Study the drawing (mm; zero at the part's minimum x, y, z) and answer. A direction names the side the tool comes from. Give positions to 0.01 mm unless a question says otherwise; leave off trailing zeros. Write each loop counter-clockwise with the first axis right and the second up, starting at its lowest first coordinate (ties: lowest second). Pieces come first, ordered by that corner, then holes. Notation, with made-up numbers: (-20, 42) -> (-16, 42) arc R18 ccw to (-16, 68) -> close; hole circle Ø6 at (15, -3.5). An arc over 180 degrees is marked (long way). Put each result on its own line as item: value. Start each with the question number.
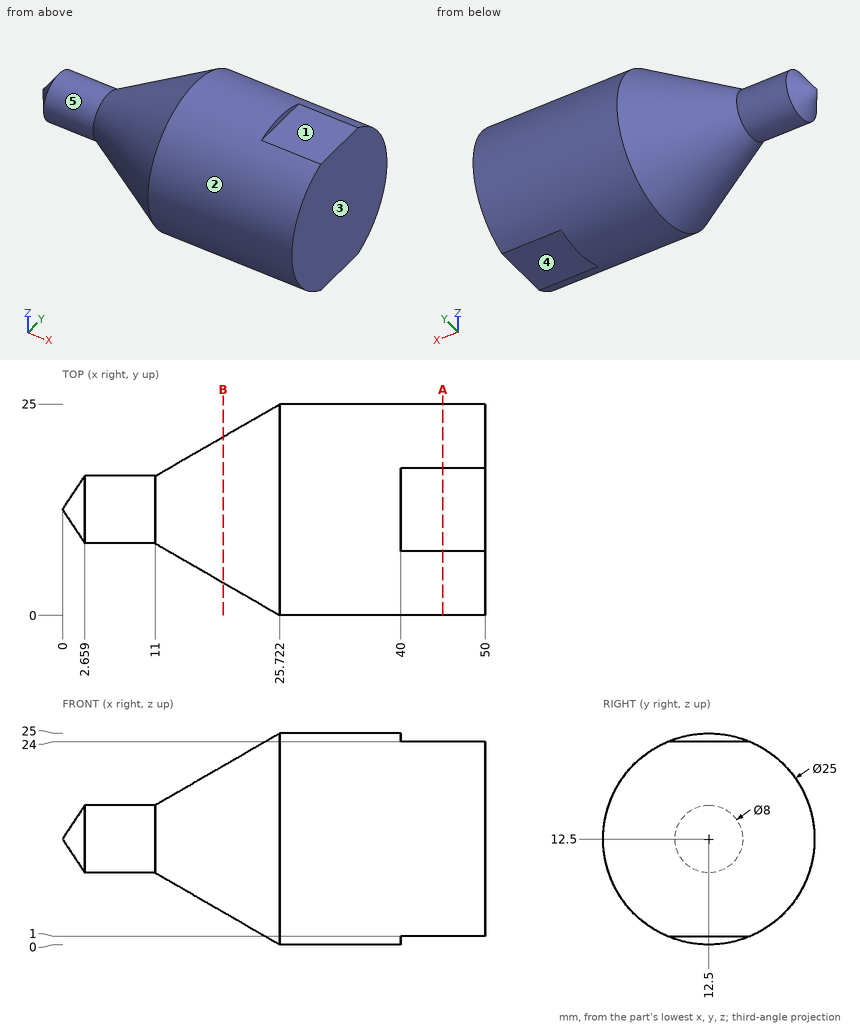
1) A cutting plane is placed at A-A on x = 45. Give the vertices of the cut face in (y, z), and give its area (3 significant figures).
2) Straight lines are drawn through the part: line 1 (Y direction, x = 37, z = 17.5) (1 decimal); line 2 (X direction, y = 1.75, z = 12.75) (1 decimal); line 3 (Y direction, x = 47.5, z = 18.25). For each, find the intervals that lie inside material, in ascending order. Write a range as [from, to].
3) For the marked faces 1, 2, 3, 4 and 5, determine the directions among +Z, -Z, +X, -X, +Y, -Y from which every point of the face is accessible in a straight line to the end or side of a thin tool.
4) Each of these flat-tipped pins is pushed along its axis until it touches: pin 1 Ø6 at (x, z) = (12, 15) entering from +Y; pin 2 Ø1.5 at (x, y) = (23, 21) entering from -Z (1 decimal); pin 3 Ø1 at (x, z) = (20, 19) entering from +Y (1 decimal); pin 4 Ø8 at (x, y) = (43, 13.5) entering from -Z. Where does it stop, or does it pass through?
5) A cutting plane is placed at B-B on x = 19. Give the vertices of the cut face in (y, z), and give its area (3 significant figures).
Results found:
1. outline: (7.6, 1) -> (17.4, 1) arc R12.5 ccw to (17.4, 24) -> (7.6, 24) arc R12.5 ccw to start
1. area: 478 mm²
2. line 1: y = [1, 24]
2. line 2: x = [22.7, 50]
2. line 3: y = [1.4, 23.6]
3. face 1: +Z, +X, +Y, -Y
3. face 2: +X, -X
3. face 3: +Z, -Z, +X, +Y, -Y
3. face 4: -Z, +X, +Y, -Y
3. face 5: -X
4. pin 1: stops at y = 18.53
4. pin 2: stops at z = 4.6
4. pin 3: stops at y = 19.6
4. pin 4: stops at z = 0
5. outline: circle Ø17.24 at (12.5, 12.5)
5. area: 233 mm²
